from build123d import *

# Parameters (mm, degrees)
SKETCH1_R           = 13.97
SKETCH1_R_2         = 12.065
BOSS_EXTRUDE1_DEPTH = 15.24
SKETCH2_R           = 13.97
SKETCH2_R_2         = 3.175
BOSS_EXTRUDE2_DEPTH = 1.27
SKETCH3_R           = 12.9286
SKETCH3_R_2         = 12.065
BOSS_EXTRUDE3_DEPTH = 6.096


with BuildPart() as part:
    # Sketch1 → Boss-Extrude1 (new body)
    with BuildSketch(Plane.XY):
        with Locations(Location((0, 0, 0), (0, 0, 180))):
            Circle(SKETCH1_R)
        with Locations(Location((0, 0, 0), (0, 0, 180))):
            Circle(SKETCH1_R_2, mode=Mode.SUBTRACT)
    extrude(amount=BOSS_EXTRUDE1_DEPTH)

    # Sketch2 → Boss-Extrude2 (add)
    with BuildSketch(Plane(origin=(0, 0, 0), x_dir=(-1, 0, 0), z_dir=(0, 0, -1))):
        Circle(SKETCH2_R)
        Circle(SKETCH2_R_2, mode=Mode.SUBTRACT)
    extrude(amount=-BOSS_EXTRUDE2_DEPTH)

    # Sketch3 → Boss-Extrude3 (add)
    with BuildSketch(Plane.XY.offset(15.24)):
        with Locations(Location((0, 0, 0), (0, 0, 180))):
            Circle(SKETCH3_R)
        with Locations(Location((0, 0, 0), (0, 0, 180))):
            Circle(SKETCH3_R_2, mode=Mode.SUBTRACT)
    extrude(amount=BOSS_EXTRUDE3_DEPTH)


solid = part.part
The listing builds one solid part. Answer for the finished solid, in the listing's coordinates (mm). A direction names the side the tool comes from. Coordinates: 2 decimals unless noted, no trailing zeros. Write each loop counter-clockwise with the first axis right and the second up, starting at its lowest first coordinate (ties: lowest second). Pieces come first, ordered by that corner, then holes. Notation, with made-up numbers: (19.5, -28) - (34.5, -28) arc R26 cw to (34.5, 11) - close; hole circle Ø9 at (86, -7.75). An arc over 180 degrees is marked (long way). Return JSON: item names as keys, results as strings.
1. The part is cut by section D-D on z = 20. Determine the outline of the cut face in (x, y) (3 decimals), then the cut area to 3 significant figures.
Final values:
{"outline": "circle Ø25.857 at (0, 0); hole circle Ø24.13 at (0, 0)", "area": "67.8 mm^2"}
2. Each of these flat-tipped pins is pushed along its axis until it touches: pin 1 Ø3 at (y, z) = (-8.5, 4) entering from -X; pin 2 Ø14 at (x, y) = (1, 1.5) entering from +Z; pin 3 Ø6 at (x, z) = (-8, 11.5) entering from +Y. Where does it stop, or does it pass through?
Final values:
{"pin 1": "x = -12.09", "pin 2": "z = 1.27", "pin 3": "y = 13.04"}
3. The part is cut by section C-C on x = -11.25. Determine the outline of the cut face in (y, z), then the cut area to 3 significant figures.
Final values:
{"outline": "(-8.28, 0) - (8.28, 0) - (8.28, 15.24) - (6.37, 15.24) - (6.37, 21.34) - (4.36, 21.34) - (4.36, 1.27) - (-4.36, 1.27) - (-4.36, 21.34) - (-6.37, 21.34) - (-6.37, 15.24) - (-8.28, 15.24) - close", "area": "155 mm^2"}
4. Which of the six approach directions +Z, -Z, +X, -X, +Y, -Y give full straight-line access (tool end or side, diameter ignored) to faces 1 (the face through (11, -6, 21.336)), 2 (the face through (-3, -3, 1.27))?
Final values:
{"face 1": "+Z, +X, -X, +Y, -Y", "face 2": "+Z"}
5. Consider line 1 along Y through (x, z) = (0, 14.75) (3 decimals); line 2 along Y through (x, z) = (0, 0.4) (3 decimals); line 3 along Z through (x, y) = (-6.5, 7.5). Determine where each line is inside the solid, lowest interval first.
Final values:
{"line 1": "-13.97 to -12.065, 12.065 to 13.97", "line 2": "-13.97 to -3.175, 3.175 to 13.97", "line 3": "0 to 1.27"}
6. The part is cut by section A-A on y = 0. Determine the outline of the cut face in (x, z) (3 decimals), then the cut area to 3 significant figures.
Final values:
{"outline": "(-13.97, 0) - (-3.175, 0) - (-3.175, 1.27) - (-12.065, 1.27) - (-12.065, 21.336) - (-12.929, 21.336) - (-12.929, 15.24) - (-13.97, 15.24) - close; (3.175, 0) - (13.97, 0) - (13.97, 15.24) - (12.929, 15.24) - (12.929, 21.336) - (12.065, 21.336) - (12.065, 1.27) - (3.175, 1.27) - close", "area": "91.2 mm^2"}
7. For a pull along X with two mould halves and no side action, classify faces 3 (the face through (-3, 3, 0)), 4 (the face through (0.69, -3.1, 0.63)), 5 (the face through (1.82, -13.85, 7.51)) as +X half, -X half, draft (parallel to the pull), parting line (faces both ways), or undercut.
Final values:
{"face 3": "draft", "face 4": "undercut", "face 5": "parting line"}
